from build123d import *

# Parameters (mm, degrees)
SKETCH_2_W            = 45.206404826
SKETCH_2_H            = 11.893552363
CUT_EXTRUDE_1_DEPTH   = 44.729866796
M3_TAPPED_HOLE1_D     = 2.5
M3_TAPPED_HOLE1_DEPTH = 15
M3_TAPPED_HOLE1_TIP   = 0.751075774
CUT_EXTRUDE_START     = -20.2
SKETCH_6_R            = 1.25
CUT_EXTRUDE_3_DEPTH   = 10
M4X0_7_TAPPED_HOLE1_D = 3.3


with BuildPart() as part:
    # Эскиз1 → Повернуть1 (revolve)
    with BuildSketch(Plane.XY, mode=Mode.PRIVATE) as revolve_1_sk:
        Polygon((-27.425, 0), (-18.75, 0), (-18.75, 8.3), (-3.5, 8.3), (-3.5, 12.2), (-17.75, 12.2), (-17.75, 20.2), (-27.425, 20.2), align=None)
    revolve(revolve_1_sk.sketch.rotate(Axis((0, 0, 0), (0, 1, 0)), 270), axis=Axis((0, 0, 0), (0, 1, 0)))

    # Эскиз2 → Вырез-Вытянуть1 (cut, through all)
    with BuildSketch(Plane.XZ):
        with Locations((0, 21.478223819)):
            Rectangle(SKETCH_2_W, SKETCH_2_H)
    extrude(amount=-CUT_EXTRUDE_1_DEPTH, mode=Mode.SUBTRACT)

    # M3 Tapped Hole1
    with Locations(Plane(origin=(0, 20.2, 0), x_dir=(1, 0, 0), z_dir=(0, 1, 0))):
        with Locations((11.435398966, 17.613394065)):
            Hole(M3_TAPPED_HOLE1_D / 2, depth=M3_TAPPED_HOLE1_DEPTH)
            with Locations((0, 0, -(M3_TAPPED_HOLE1_DEPTH + M3_TAPPED_HOLE1_TIP / 2))):  # 118° drill point
                Cone(0, M3_TAPPED_HOLE1_D / 2, M3_TAPPED_HOLE1_TIP, mode=Mode.SUBTRACT)

    # Эскиз6 → Вырез-Вытянуть3 (cut)
    with BuildSketch(Plane.XZ.offset(CUT_EXTRUDE_START)):
        with Locations(Location((20.561874638, -12.118552363, 0), (0, 0, 270))):
            Circle(SKETCH_6_R)
        with Locations(Location((-8.822328368, -22.500922696, 0), (0, 0, 270))):
            Circle(SKETCH_6_R)
        with Locations(Location((-24.522435774, -6.541065947, 0), (0, 0, 270))):
            Circle(SKETCH_6_R)
    extrude(amount=CUT_EXTRUDE_3_DEPTH, mode=Mode.SUBTRACT)

    # M4x0.7 Tapped Hole1 (through all)
    with Locations(Plane(origin=(0, 0, 0), x_dir=(-1, 0, 0), z_dir=(0, -1, 0))):
        with Locations((-21.909616243, -6.997765079)):
            Hole(M4X0_7_TAPPED_HOLE1_D / 2)


solid = part.part
Input: part model. Units: mm. Frame: model coordinates. A direction names the side the tool comes from. Coordinates: 2 decimals unless noted, no trailing zeros. Loops run counter-clockwise (first coordinate to the right, second up) from the corner with the lowest first, then second, coordinate; pieces in that order, holes last.
Q1. Material intervals for line 1 (Y direction, x = 7, z = 4); line 2 (X direction, y = 7, z = 4); line 3 (X direction, y = 11, z = -13), sorted ascending.
Q2. Contact query for flat-ended pins moving along their axis: pin 1 (6 mm diameter, centred on x = -11, z = -4.5, fed in from +Y); pin 2 (4 mm diameter, centred on x = 0, z = 0, fed in from -Y); pin 3 (17 mm diameter, centred on x = -1.5, z = -9, fed in from -Y); pin 4 (3 mm diameter, centred on y = 16, z = -21, fed in from +X). Output: stop coordinate, or through.
Q3. Cut plane D-D (y = 2). Output: boundary loops of the cut face in (x, z) (3 decimals).
Q4. Cut plane B-B (z = 0). Output: boundary loops of the cut face in (x, y) (3 decimals), then the cut area to 3 significant figures.
Q5. Set-up query: faces 1 (the face through (-25, 10.2, -7)), 2 (the face through (0, 0, -20)), 3 (the face through (0.67, 4.21, -18.74)). Return all of +Z, -Z, +X, -X, +Y, -Y with unobstructed straight access to the full face (end or side cutting, diameter ignored); none if empty.
Q6. Cut plane A-A (x = 0). Output: boundary loops of the cut face in (y, z) (3 decimals), then the cut area to 3 significant figures.
Q7. Cut plane C-C (y = 17.25). Output: boundary loops of the cut face in (x, z) (3 decimals).
Working result:
1. line 1: y = 8.3 to 12.2
1. line 2: x = -27.13 to -18.32, 18.32 to 27.13
1. line 3: x = -24.15 to 19.68, 21.45 to 24.15
2. pin 1: stops at y = 12.2
2. pin 2: passes through
2. pin 3: stops at y = 8.3
2. pin 4: stops at x = 19.28
3. outline: (-22.603, 15.531) arc R27.425 ccw (long way) to (22.603, 15.531) - (10.504, 15.531) arc R18.75 cw (long way) to (-10.504, 15.531) - close; hole circle Ø3.3 at (21.91, 6.998)
4. outline: (-27.425, 0) - (-18.75, 0) - (-18.75, 8.3) - (-3.5, 8.3) - (-3.5, 12.2) - (-17.75, 12.2) - (-17.75, 20.2) - (-27.425, 20.2) - close; (3.5, 8.3) - (18.75, 8.3) - (18.75, 0) - (27.425, 0) - (27.425, 20.2) - (17.75, 20.2) - (17.75, 12.2) - (3.5, 12.2) - close
4. area: 485 mm2
5. face 1: +Y
5. face 2: +Z, -Z, +X, -X, -Y
5. face 3: -Y
6. outline: (0, -27.425) - (20.2, -27.425) - (20.2, -17.75) - (12.2, -17.75) - (12.2, -3.5) - (8.3, -3.5) - (8.3, -18.75) - (0, -18.75) - close; (8.3, 3.5) - (12.2, 3.5) - (12.2, 15.531) - (8.3, 15.531) - close
6. area: 290 mm2
7. outline: (-22.603, 15.531) arc R27.425 ccw (long way) to (22.603, 15.531) - (8.593, 15.531) arc R17.75 cw (long way) to (-8.593, 15.531) - close; hole circle Ø2.5 at (-24.522, -6.541); hole circle Ø2.5 at (-8.822, -22.501); hole circle Ø2.5 at (11.435, -17.613); hole circle Ø2.5 at (20.562, -12.119); hole circle Ø3.3 at (21.91, 6.998)
